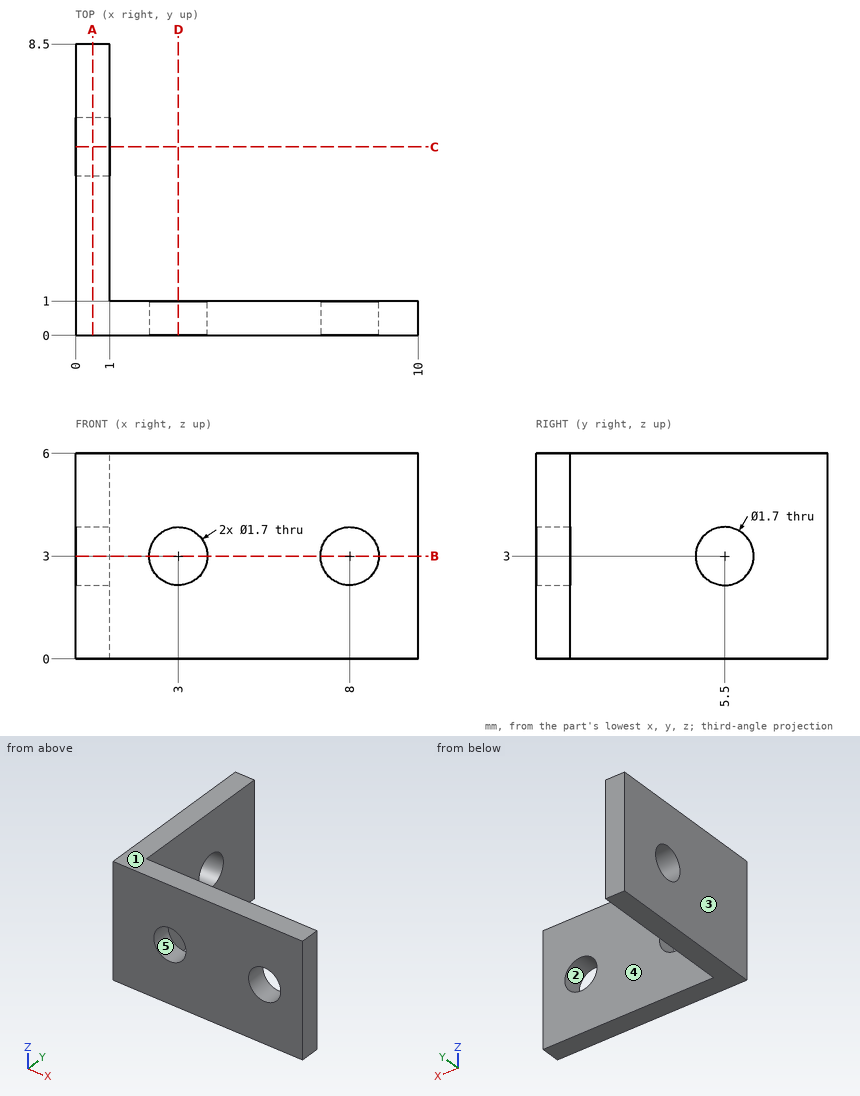
Input: dimensioned drawing with shaded views. Units: mm. Origin: part minimum x, y, z. A direction names the side the tool comes from. Coordinates: 2 decimals unless noted, no trailing zeros. Order: outer loops, then holes, each group sorted by start corner. A loop starts at its lowest first (then second) coordinate and runs counter-clockwise, first axis right, second up. Notation, with made-up numbers: (55.25, -39.75) - (103.25, -39.75) arc R26 cw to (103.25, -13.75) - close; hole circle Ø3 at (61.5, -39). An arc over 180 degrees is marked (long way). One line per item, written item: value.
1) Mould query, pull axis Z, two halves, no side actions, for the marked faces 1, 2 and 3. Classes: released by +Z, released by -Z, zero draft, split by the parting line, or undercut.
Computed values:
face 1: released by +Z
face 2: undercut
face 3: zero draft
2) Reachability of the marked faces 4 and 5 from +Z, -Z, +X, -X, +Y, -Y: full face, straight path, thin tool, end or side. Return the list, or none.
Computed values:
face 4: +Z, -Z, +X, +Y
face 5: +Y, -Y
3) Cut plane C-C on y = 5.5. Output: boundary loops of the cut face in (x, z), plus the area to 3 significant figures.
Computed values:
outline: (0, 0) - (1, 0) - (1, 2.15) - (0, 2.15) - close; (0, 3.85) - (1, 3.85) - (1, 6) - (0, 6) - close
area: 4.30 mm^2
4) Cut plane A-A on x = 0.5. Output: boundary loops of the cut face in (y, z), plus the area to 3 significant figures.
Computed values:
outline: (0, 0) - (8.5, 0) - (8.5, 6) - (0, 6) - close; hole circle Ø1.7 at (5.5, 3)
area: 48.7 mm^2
5) Cut plane B-B on z = 3. Output: boundary loops of the cut face in (x, y), plus the area to 3 significant figures.
Computed values:
outline: (0, 0) - (2.15, 0) - (2.15, 1) - (1, 1) - (1, 4.65) - (0, 4.65) - close; (0, 6.35) - (1, 6.35) - (1, 8.5) - (0, 8.5) - close; (3.85, 0) - (7.15, 0) - (7.15, 1) - (3.85, 1) - close; (8.85, 0) - (10, 0) - (10, 1) - (8.85, 1) - close
area: 12.4 mm^2
6) Contact query for flat-ended pins moving along their axis: pin 1 (3 mm diameter, centred on y = 6, z = 2, fed in from +X); pin 2 (3 mm diameter, centred on x = 5.5, z = 2.5, fed in from +Y). Output: stop coordinate, or through.
Computed values:
pin 1: stops at x = 1
pin 2: stops at y = 1
7) Ray query, line 1 (Z direction, x = 0.6, y = 5.5); line 2 (X direction, y = 7.5, z = 4). Return the intervals inside material, ascending. Write a range as [from, to].
Computed values:
line 1: z = [0, 2.15], [3.85, 6]
line 2: x = [0, 1]
